Read the model definition and answer for the solid it produces. Units are mm, in the model's axes. A direction names the side the tool comes from. Coordinates: 2 decimals unless noted, no trailing zeros. Loops run counter-clockwise (first coordinate to the right, second up) from the corner with the lowest first, then second, coordinate; pieces in that order, holes last. Notation, with made-up numbers: (64, 51) -> (116, 51) arc R20 ccw to (116, 60) -> close; hole circle Ø7 at (-7.5, 29). An arc over 180 degrees is marked (long way). Answer as a JSON object with one key per item and string values. Group by question number.
1) Section C-C, the plane z = 0 is taken. Give the vertices of the cut face in (x, y), plus the area to 3 significant figures.
2) Section D-D, the plane y = -16 is taken. Give the vertices of the cut face in (x, z).
3) Flat-ended cylindrical pins translate along their axes: P1, Ø1, axis at x = 3, y = -1.5, coming from the -Z side; P2, Ø3, axis at y = -10, z = -13.5, coming from the +X side; P3, Ø2, axis at x = -3, y = -6.5, coming from the +Z side. Find the tip coordinate at first contact, or state that the pin passes through.
4) Section B-B, the plane y = 1 is taken. Give the vertices of the cut face in (x, z).
5) Section A-A, the plane x = 0 is taken. Give the vertices of the cut face in (y, z), plus the area to 3 significant figures.
6) Which of the six approach directions +Z, -Z, +X, -X, +Y, -Y give full straight-line access (tool end or side, diameter ignored) to faces 5 (the face through (6.429, -17.44, -8.385)), 6 (the face through (-8, 17.78, -13))?
7) Consider probe 1 along Y at (x, z) = (14, 3); probe 2 along X at (y, z) = (15.95, 0); probe 3 along Z at (x, y) = (-3, 16). Determine where each line is inside the solid, lowest interval first. Write a range as [from, to].
8) Determine the mould class of faces 1 (the face through (-5.691, 16.528, 13.726)), 2 (the face through (12, 7.874, -12)), 3 (the face through (16.08, 10.56, -3.57)), 4 (the face through (0, 15.24, 0)) for opening direction Y: released by +Y, released by -Y, zero draft, split by the parting line, or undercut.
from build123d import *

# Parameters (mm, degrees)
SKETCH2_R          = 14.859
CUT_EXTRUDE1_DEPTH = 2.54


with BuildPart() as part:
    # Sketch1 → Revolve1 (revolve)
    with BuildSketch(Plane(origin=(0, 0, 0), x_dir=(0, 0, -1), z_dir=(1, 0, 0))):
        Polygon((0, 17.78), (-17.399, 17.78), (-16.129, 7.874), (-17.399, 7.874), (-17.399, 0), (-13.1064, 0), (-13.1064, -14.478), (-10.5664, -14.478), (-10.5664, -20.32), (0, -20.32), align=None)
    revolve(axis=Axis((0, 17.78, 0), (0, -1, 0)))

    # Sketch2 → Cut-Extrude1 (cut)
    with BuildSketch(Plane(origin=(0, 17.78, 0), x_dir=(1, 0, 0), z_dir=(0, 1, 0))):
        with Locations(Location((0, 0, 0), (0, 0, 270))):
            Circle(SKETCH2_R)
    extrude(amount=-CUT_EXTRUDE1_DEPTH, mode=Mode.SUBTRACT)


solid = part.part
Determined:
{
 "1": {"outline": "(-17.4, 0) -> (-13.11, 0) -> (-13.11, -14.48) -> (-10.57, -14.48) -> (-10.57, -20.32) -> (10.57, -20.32) -> (10.57, -14.48) -> (13.11, -14.48) -> (13.11, 0) -> (17.4, 0) -> (17.4, 7.87) -> (16.13, 7.87) -> (17.4, 17.78) -> (14.86, 17.78) -> (14.86, 15.24) -> (-14.86, 15.24) -> (-14.86, 17.78) -> (-17.4, 17.78) -> (-16.13, 7.87) -> (-17.4, 7.87) -> close", "area": "1,030 mm²"},
 "2": {"outline": "circle Ø21.13 at (0, 0)"},
 "3": {"P1": "z = -12.87", "P2": "x = 5.27", "P3": "z = 12.95"},
 "4": {"outline": "circle Ø34.8 at (0, 0)"},
 "5": {"outline": "(-20.32, -10.57) -> (-14.48, -10.57) -> (-14.48, -13.11) -> (0, -13.11) -> (0, -17.4) -> (7.87, -17.4) -> (7.87, -16.13) -> (17.78, -17.4) -> (17.78, -14.86) -> (15.24, -14.86) -> (15.24, 14.86) -> (17.78, 14.86) -> (17.78, 17.4) -> (7.87, 16.13) -> (7.87, 17.4) -> (0, 17.4) -> (0, 13.11) -> (-14.48, 13.11) -> (-14.48, 10.57) -> (-20.32, 10.57) -> close", "area": "1,030 mm²"},
 "6": {"face 5": "-Y", "face 6": "+Z, -Z, +X, -X, +Y"},
 "7": {"probe 1": "[0, 15.24]", "probe 2": "[-17.16, -14.86], [14.86, 17.16]", "probe 3": "[-16.91, -14.55], [14.55, 16.91]"},
 "8": {"face 1": "zero draft", "face 2": "undercut", "face 3": "undercut", "face 4": "released by +Y"}
}
